CAD build for the part. Positions are in the model's coordinates, mm. Face numbers are marked on the shaded views. A direction names the side the tool comes from. Round coordinates to 2 decimals unless told otherwise and drop trailing zeros. Order: outer loops, then holes, each group sorted by start corner. A loop starts at its lowest first (then second) coordinate and runs counter-clockwise, first axis right, second up.
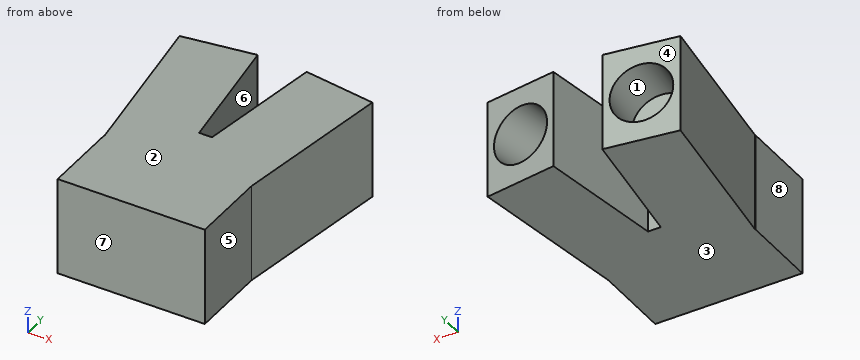
```python
from build123d import *

# Parameters (mm, degrees)
F1_DEPTH = 20
F2_R     = 6.0518975937
F3_DEPTH = 10
F4_R     = 6
F5_DEPTH = 10


with BuildPart() as f1:
    # F0 (on Top) → F1 (new body)
    with BuildSketch(Plane.XY):
        Polygon((-5, 35), (-19.7, 32.9), (-15, 0), (-15.0675689802, 0), (-15.0675689802, -15.7475546002), (15, -15.7475546002), (15, 0), (19.7, 32.9), (5, 35), (1.3167639755, 9.2173478283), (-1.3167639755, 9.2173478283), align=None)
    extrude(amount=F1_DEPTH)

    # F2 (on face) → F3 (cut)
    with BuildSketch(Plane(origin=(-5, 35, 0), x_dir=(-0.9899494937, -0.1414213562, 0), z_dir=(-0.1414213562, 0.9899494937, 0))):
        with Locations((7.4246212025, 10)):
            Circle(F2_R)
    extrude(amount=-F3_DEPTH, mode=Mode.SUBTRACT)

    # F4 (on face) → F5 (cut)
    with BuildSketch(Plane(origin=(5, 35, 0), x_dir=(-0.9899494937, 0.1414213562, 0), z_dir=(0.1414213562, 0.9899494937, 0))):
        with Locations((-7.4246212025, 10)):
            Circle(F4_R)
    extrude(amount=-F5_DEPTH, mode=Mode.SUBTRACT)


solid = f1.part
```
1. Cut at C-C, the plane x = -4. Write the cut outline in (y, z), and give its area (3 significant figures).
2. Pin check, flat tips, straight feed: P1, Ø1.5, axis at y = 19, z = 11, coming from the -X side; P2, Ø10, axis at y = -3.5, z = 15, coming from the +X side; P3, Ø8, axis at y = -9.5, z = 10, coming from the -X side. Stop position of each tip, or through.
3. Drill centre lines: line 1 (Z direction, x = -12, y = 29); line 2 (X direction, y = 26.5, z = 13); line 3 (X direction, y = 28, z = 12.75). Where is each one in solid material? Low to high.
4. Cut at D-D, the plane y = -6.5. Write the cut outline in (x, z), and give its area (3 significant figures).
5. Cut at A-A, the plane y = 17. Write the cut outline in (x, z).
6. Tool access for the marked faces 4, 5, 6, 7 and 8: list every direction of +Z, -Z, +X, -X, +Y, -Y with a clear straight run to the whole face (end or side of a thin tool).
7. Cut at B-B, the plane z = 1.75. Write the cut outline in (x, y), and give its area (3 significant figures).
8. Mould opens along Z. For the marked faces 1, 2 and 3 say: released by +Z, released by -Z, zero draft, split by the parting line, or undercut.
Outcome:
1. outline: (-15.75, 0) - (28, 0) - (28, 20) - (-15.75, 20) - close
1. area: 875 mm2
2. P1: stops at x = -17.82
2. P2: stops at x = 15.21
2. P3: stops at x = -15.07
3. line 1: z = 0 to 3.96, 16.04 to 20
3. line 2: x = -18.79 to -16.6, -5.98 to -3.79, 3.79 to 6.04, 16.53 to 18.79
3. line 3: x = -19 to -16.95, -6.05 to -4, 4 to 6.11, 16.89 to 19
4. outline: (-15.07, 0) - (15, 0) - (15, 20) - (-15.07, 20) - close
4. area: 601 mm2
5. outline: (-17.43, 0) - (-2.43, 0) - (-2.43, 20) - (-17.43, 20) - close; (2.43, 0) - (17.43, 0) - (17.43, 20) - (2.43, 20) - close
6. face 4: +Z, -Z, -X, +Y
6. face 5: +Z, -Z, +X, -Y
6. face 6: +Z, -Z, +Y
6. face 7: +Z, -Z, +X, -X, -Y
6. face 8: +Z, -Z, -X, -Y
7. outline: (-19.7, 32.9) - (-15, 0) - (-15.07, 0) - (-15.07, -15.75) - (15, -15.75) - (15, 0) - (19.7, 32.9) - (5, 35) - (1.32, 9.22) - (-1.32, 9.22) - (-5, 35) - close
7. area: 1,500 mm2
8. face 1: undercut
8. face 2: released by +Z
8. face 3: released by -Z
